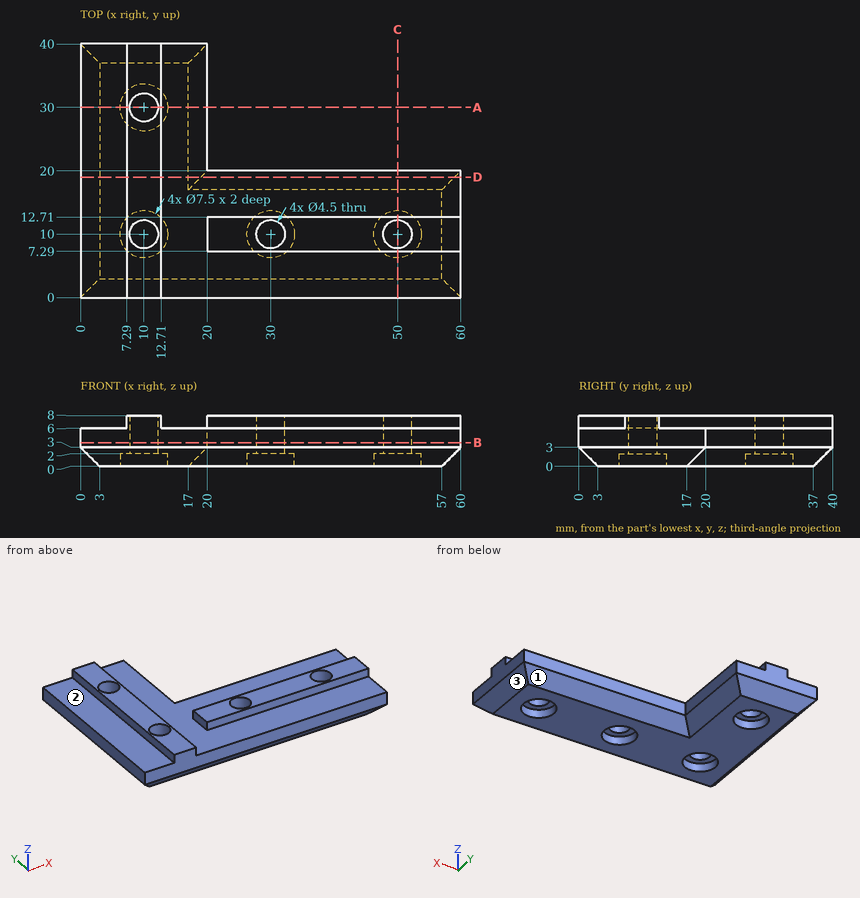
Could you check a few things on this drawing? It's one solid part, dimensions in mm from its lowest x, y, z. A direction names the side the tool comes from. Round coordinates to 2 decimals unless told otherwise and drop trailing zeros. Order: outer loops, then holes, each group sorted by start corner. A loop starts at its lowest first (then second) coordinate and runs counter-clockwise, first axis right, second up.
Q1. Please list where these lines run through material, in increasing order: probe 1 along Y at (x, z) = (50, 4.5); probe 2 along X at (y, z) = (19, 7.25); probe 3 along Y at (x, z) = (10, 1.45).
Geometry says:
probe 1: y = 0 to 7.75, 12.25 to 20
probe 2: x = 7.29 to 12.71
probe 3: y = 1.55 to 6.25, 13.75 to 26.25, 33.75 to 38.45
Q2. Imagine slicing it at B-B, the plane z = 3.75. List the corners of the cut face in (x, y) for me.
Geometry says:
outline: (0, 0) - (60, 0) - (60, 20) - (20, 20) - (20, 40) - (0, 40) - close; hole circle Ø4.5 at (10, 10); hole circle Ø4.5 at (10, 30); hole circle Ø4.5 at (30, 10); hole circle Ø4.5 at (50, 10)
Q3. Imagine slicing it at D-D, the plane y = 19. List the corners of the cut face in (x, z) for me, then the cut area to 3 significant figures.
Geometry says:
outline: (0, 3) - (3, 0) - (17, 0) - (19, 2) - (59, 2) - (60, 3) - (60, 6) - (12.71, 6) - (12.71, 8) - (7.29, 8) - (7.29, 6) - (0, 6) - close
area: 282 mm2
Q4. Which directions (+Z, -Z, +X, -X, +Y, -Y) give clear straight access to the entire face, cutting with the end or side of a thin tool? Please do the marked faces 1, 2 and 3.
Geometry says:
face 1: -Z, +X, +Y
face 2: +Z, -X, +Y, -Y
face 3: -Z, +X, +Y, -Y
Q5. Imagine slicing it at A-A, the plane y = 30. List the corners of the cut face in (x, z) for me, then the cut area to 3 significant figures.
Geometry says:
outline: (0, 3) - (3, 0) - (6.25, 0) - (6.25, 2) - (7.75, 2) - (7.75, 8) - (7.29, 8) - (7.29, 6) - (0, 6) - close; (12.25, 2) - (13.75, 2) - (13.75, 0) - (17, 0) - (20, 3) - (20, 6) - (12.71, 6) - (12.71, 8) - (12.25, 8) - close
area: 79.8 mm2
Q6. I'm going to push flat-ended pins straight in: P1, Ø0.6, axis at y = 29, z = 6.5, coming from the -X side; P2, Ø0.6, axis at y = 20.5, z = 7, coming from the +X side; P3, Ø1, axis at x = 49, z = 7, coming from the +Y side; P4, Ø3.5, axis at x = 50, y = 10, coming from the -Z side. Where does each tip first touch, or does it pass through?
Geometry says:
P1: stops at x = 7.29
P2: stops at x = 12.71
P3: stops at y = 12.71
P4: passes through
